```python
from build123d import *

# Parameters (mm, degrees)
EXTRUDE_START   = 20
SKETCH_1_R      = 4
EXTRUDE_1_DEPTH = 5


with BuildPart() as part:
    # ｽｹｯﾁ1 → ﾎﾞｽ - 押し出し1 (new body)
    with BuildSketch(Plane.XY.offset(EXTRUDE_START)):
        Polygon((0, 22), (16, 22), (35.5, 54), (35.5, 86), (7.5, 86), (0, 38), align=None)
        with Locations((8, 30)):
            Circle(SKETCH_1_R, mode=Mode.SUBTRACT)
    extrude(amount=EXTRUDE_1_DEPTH)


solid = part.part
```
Here's how the part is built. I have some questions about the finished solid (model axes, mm). Coordinates: 2 decimals unless noted, no trailing zeros. Order: outer loops, then holes, each group sorted by start corner. A loop starts at its lowest first (then second) coordinate and runs counter-clockwise, first axis right, second up. Notation, with made-up numbers: M -7,-24 L -3,-24 A20 cw -3,-14 Z; hole C 41.25,60.25 d5. An arc over 180 degrees is marked long. Answer as a JSON object with one key per item and string values. Group by question number.
(1) If we mould it in two halves opening along Y, with no side actions, what happens to faces 1 (the face through (18, 54, 20)), 2 (the face through (8, 22, 22)), 3 (the face through (7.479, 33.966, 22.465))? For each: released by +Y, released by -Y, zero draft, split by the parting line, or undercut.
(2) Suppose I cut it at B-B, the plane y = 30. Please give me the cut outline in (x, z) (3 decimals).
(3) Suppose I cut it at C-C, the plane x = 27. Please give me the cut outline in (y, z).
(4) Suppose I cut it at A-A, the plane z = 23.8. Please give me the cut outline in (x, y).
(5) Suppose I cut it at D-D, the plane y = 63. Please give me the cut outline in (x, z), then the cut area to 3 significant figures.
(6) I need wall thicknesses on probe 1 along Y at (x, z) = (8, 21); probe 2 along Y at (x, z) = (10.5, 22); probe 3 along Y at (x, z) = (30.5, 24.7). Which ranges of each line are inside material? Lowest first, please.
Values found:
{
 "1": {"face 1": "zero draft", "face 2": "released by -Y", "face 3": "undercut"},
 "2": {"outline": "M 0,20 L 4,20 L 4,25 L 0,25 Z; M 12,20 L 20.875,20 L 20.875,25 L 12,25 Z"},
 "3": {"outline": "M 40.05,20 L 86,20 L 86,25 L 40.05,25 Z"},
 "4": {"outline": "M 0,22 L 16,22 L 35.5,54 L 35.5,86 L 7.5,86 L 0,38 Z; hole C 8,30 d8"},
 "5": {"outline": "M 3.91,20 L 35.5,20 L 35.5,25 L 3.91,25 Z", "area": "158 mm^2"},
 "6": {"probe 1": "y = 22 to 26, 34 to 86", "probe 2": "y = 22 to 26.88, 33.12 to 86", "probe 3": "y = 45.79 to 86"}
}
